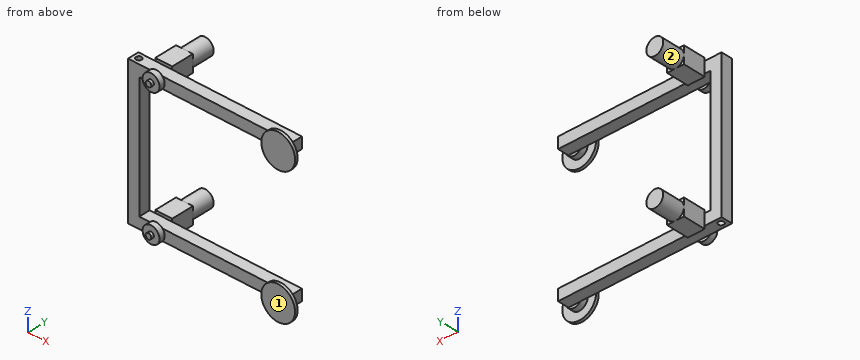
```python
from build123d import *

# Parameters (mm, degrees)
BOSS_EXTRUDE1_DEPTH     = 25.4
SKETCH3_W               = 38.1
SKETCH3_H               = 38.1
BOSS_EXTRUDE2_DEPTH     = 50.8
SKETCH4_R               = 19.05
BOSS_EXTRUDE3_DEPTH     = 50.8
LPATTERN1_COUNT         = 2
LPATTERN1_PITCH         = 304.8
SKETCH5_R               = 19.05
BOSS_EXTRUDE4_DEPTH     = 12.7
SKETCH6_R               = 6.35
BOSS_EXTRUDE5_DEPTH     = 6.35
LPATTERN2_COUNT         = 2
LPATTERN2_PITCH         = 304.8
SKETCH7_R               = 19.05
BOSS_EXTRUDE6_DEPTH     = 12.7
SKETCH8_R               = 38.1
BOSS_EXTRUDE7_DEPTH     = 6.35
LPATTERN3_COUNT         = 2
LPATTERN3_PITCH         = 304.8
CUT_EXTRUDE1_DEPTH      = 546.889568885
CUT_EXTRUDE1_DEPTH_BACK = 546.889568885
SKETCH9_R               = 6.35


with BuildPart() as part:
    # Sketch1 → Boss-Extrude1 (new body)
    with BuildSketch(Plane(origin=(0, 0, 0), x_dir=(1, 0, 0), z_dir=(0, 1, 0))):
        Polygon((0, 0), (0, 166.346037736), (368.827169811, 166.346037736), (368.827169811, 140.946037736), (25.4, 140.946037736), (25.4, -138.453962264), (368.827169811, -138.453962264), (368.827169811, -163.853962264), (0, -163.853962264), align=None)
    extrude(amount=BOSS_EXTRUDE1_DEPTH)

    # Sketch3 → Boss-Extrude2 (add)
    with BuildSketch(Plane(origin=(0, 25.4, 0), x_dir=(1, 0, 0), z_dir=(0, 1, 0))):
        with Locations((57.15, -151.153962264)):
            Rectangle(SKETCH3_W, SKETCH3_H)
    boss_extrude2 = extrude(amount=BOSS_EXTRUDE2_DEPTH)

    # Sketch4 → Boss-Extrude3 (add)
    with BuildSketch(Plane(origin=(0, 76.2, 0), x_dir=(1, 0, 0), z_dir=(0, 1, 0))):
        with Locations(Location((57.15, -151.153962264, 0), (0, 0, 270))):
            Circle(SKETCH4_R)
    boss_extrude3 = extrude(amount=BOSS_EXTRUDE3_DEPTH)

    # LPattern1: Boss-Extrude2, Boss-Extrude3 ×2
    with Locations(*[(0, 0, -i * LPATTERN1_PITCH) for i in range(1, LPATTERN1_COUNT)]):
        add(boss_extrude2)
        add(boss_extrude3)

    # Sketch5 → Boss-Extrude4 (add)
    with BuildSketch(Plane.XZ):
        with Locations(Location((63.5, 151.153962264, 0), (0, 0, 41.810314896))):
            Circle(SKETCH5_R)
    boss_extrude4 = extrude(amount=BOSS_EXTRUDE4_DEPTH)

    # Sketch6 → Boss-Extrude5 (add)
    with BuildSketch(Plane.XZ.offset(12.7)):
        with Locations(Location((63.5, 151.153962264, 0), (0, 0, 270))):
            Circle(SKETCH6_R)
    boss_extrude5 = extrude(amount=BOSS_EXTRUDE5_DEPTH)

    # LPattern2: Boss-Extrude4, Boss-Extrude5 ×2
    with Locations(*[(0, 0, -i * LPATTERN2_PITCH) for i in range(1, LPATTERN2_COUNT)]):
        add(boss_extrude4)
        add(boss_extrude5)

    # Sketch7 → Boss-Extrude6 (add)
    with BuildSketch(Plane.XZ):
        with Locations(Location((356.127169811, 151.153962264, 0), (0, 0, 138.189685104))):
            Circle(SKETCH7_R)
    boss_extrude6 = extrude(amount=BOSS_EXTRUDE6_DEPTH)

    # Sketch8 → Boss-Extrude7 (add)
    with BuildSketch(Plane.XZ.offset(12.7)):
        with Locations(Location((356.127169811, 151.153962264, 0), (0, 0, 270))):
            Circle(SKETCH8_R)
    boss_extrude7 = extrude(amount=BOSS_EXTRUDE7_DEPTH)

    # LPattern3: Boss-Extrude6, Boss-Extrude7 ×2
    with Locations(*[(0, 0, -i * LPATTERN3_PITCH) for i in range(1, LPATTERN3_COUNT)]):
        add(boss_extrude6)
        add(boss_extrude7)

    # Sketch9 → Cut-Extrude1 (cut, two sides: drawn at the far end of the back side and taken through both)
    with BuildSketch(Plane.XY.offset(163.853962264).offset(-CUT_EXTRUDE1_DEPTH_BACK)):
        with Locations(Location((12.7, 12.7, 0), (0, 0, 180))):
            Circle(SKETCH9_R)
    extrude(amount=CUT_EXTRUDE1_DEPTH + CUT_EXTRUDE1_DEPTH_BACK, mode=Mode.SUBTRACT)


solid = part.part
```
Work out the finished part from the listing and answer in its coordinate system (mm). Face numbers are marked on the shaded views. A direction names the side the tool comes from. Give positions to 0.01 mm unless a question says otherwise; leave off trailing zeros. Order: outer loops, then holes, each group sorted by start corner. A loop starts at its lowest first (then second) coordinate and runs counter-clockwise, first axis right, second up.
1. Section C-C, the plane x = 12.7 is taken. Determine the outline of the cut face in (y, z).
Result sheet:
outline: (0, -166.35) - (6.35, -166.35) - (6.35, 163.85) - (0, 163.85) - close; (19.05, -166.35) - (25.4, -166.35) - (25.4, 163.85) - (19.05, 163.85) - close
2. Section B-B, the plane y = 12.7 is taken. Determine the outline of the cut face in (x, z).
Result sheet:
outline: (0, -166.35) - (6.35, -166.35) - (6.35, 163.85) - (0, 163.85) - close; (19.05, -166.35) - (368.83, -166.35) - (368.83, -140.95) - (25.4, -140.95) - (25.4, 138.45) - (368.83, 138.45) - (368.83, 163.85) - (19.05, 163.85) - close
3. For the marked faces 1 and 2, determine the directions among +Z, -Z, +X, -X, +Y, -Y from which every point of the face is accessible in a straight line to the end or side of a thin tool.
Result sheet:
face 1: +Z, -Z, +X, -X, -Y
face 2: +Y
4. Section A-A, the plane x = 158.5 is taken. Determine the outline of the cut face in (y, z), and give its area (3 significant figures).
Result sheet:
outline: (0, -166.35) - (25.4, -166.35) - (25.4, -140.95) - (0, -140.95) - close; (0, 138.45) - (25.4, 138.45) - (25.4, 163.85) - (0, 163.85) - close
area: 1,290 mm2
5. Each of these flat-tipped pins is pushed along its axis until it touches: P1, Ø11.5, axis at x = 50, y = 58, coming from the +Z side; P2, Ø6, axis at x = 136, z = 147, coming from the +Y side; P3, Ø5, axis at x = 49.5, z = 135.5, coming from the -Y side. Where does it stop, or does it pass through?
Result sheet:
P1: stops at z = 170.2
P2: stops at y = 25.4
P3: stops at y = -12.7
6. Straight lines are drawn through the part: L1, parallel to Y at x = 12.7, z = -41; L2, parallel to X at y = 12, z = -32; L3, parallel to Z at x = 114.5, y = 2.5. For each, find the intervals that lie inside material, in ascending order.
Result sheet:
L1: y = 0 to 6.35, 19.05 to 25.4
L2: x = 0 to 6.39, 19.01 to 25.4
L3: z = -166.35 to -140.95, 138.45 to 163.85
7. Section D-D, the plane z = -43.5 is taken. Determine the outline of the cut face in (x, y), and give its area (3 significant figures).
Result sheet:
outline: (0, 0) - (25.4, 0) - (25.4, 25.4) - (0, 25.4) - close; hole circle Ø12.7 at (12.7, 12.7)
area: 518 mm2
